Design review of the part shown in the three views and the two pictorial views. Dimensions are in mm from the part's minimum x, y and z. A direction names the side the tool comes from. Round coordinates to 2 decimals unless told otherwise and drop trailing zeros. Write each loop counter-clockwise with the first axis right and the second up, starting at its lowest first coordinate (ties: lowest second). Pieces come first, ordered by that corner, then holes. Notation, with made-up numbers: (-14, 49) - (33, 49) arc R6 cw to (33, 54) - close; hole circle Ø11 at (-23, 17.5). An arc over 180 degrees is marked (long way). One line per item, written item: value. Start each with the question number.
Q1. Clearance check with flat-ended pins moving along their axes: pin 1 Ø1.5 at (x, y) = (6.5, 1) entering from +Z; pin 2 Ø1 at (x, z) = (1.5, 3) entering from +Y; pin 3 Ø0.9 at (x, y) = (7.5, 2) entering from -Z; pin 4 Ø0.9 at (y, z) = (2, 1.5) entering from +X. State where each tip first meets the part, or that it passes through.
Q2. Mouldability with a two-part tool opening along X and no side actions: class the marked faces 4, 5, 6 and 7 as +X half, -X half, draft (parallel to the pull), parting line (faces both ways), or undercut.
Q3. Add section A-A on x = 4.2. Write out the cut boundary in (y, z), and give its area (3 significant figures).
Q4. Add section D-D on x = 1.5. Write out the cut boundary in (y, z).
Q5. Tool access review of the marked faces 1, 2 and 3: name each direction out of +Z, -Z, +X, -X, +Y, -Y from which nothing blocks a thin tool from reaching the whole face with its end or side.
Q6. Add section C-C on z = 12. Write out the cut boundary in (x, y), and give its area (3 significant figures).
Q7. Add section B-B on y = 1.15. Write out the cut boundary in (x, z).
Q8. For probe 1 along Z at (x, y) = (4.25, 1); probe 2 along Z at (x, y) = (6.5, 2.1); probe 3 along X at (y, z) = (1.65, 5), list the stretches that pass through material, from the lowest coordinate up.
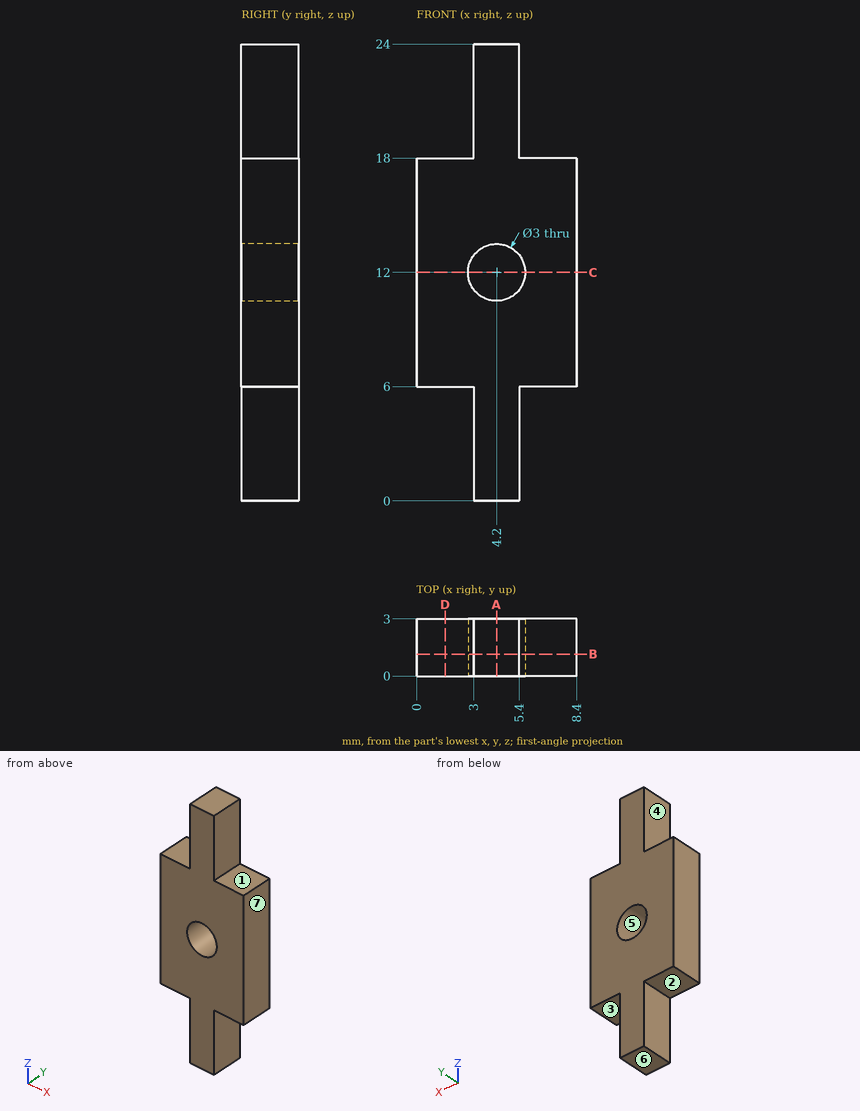
Result set:
1. pin 1: stops at z = 18
1. pin 2: passes through
1. pin 3: stops at z = 6
1. pin 4: stops at x = 5.4
2. face 4: -X half
2. face 5: undercut
2. face 6: draft
2. face 7: +X half
3. outline: (0, 0) - (3, 0) - (3, 10.5) - (0, 10.5) - close; (0, 13.5) - (3, 13.5) - (3, 24) - (0, 24) - close
3. area: 63.0 mm^2
4. outline: (0, 6) - (3, 6) - (3, 18) - (0, 18) - close
5. face 1: +Z, +X, +Y, -Y
5. face 2: -Z, -X, +Y, -Y
5. face 3: -Z, +X, +Y, -Y
6. outline: (0, 0) - (2.7, 0) - (2.7, 3) - (0, 3) - close; (5.7, 0) - (8.4, 0) - (8.4, 3) - (5.7, 3) - close
6. area: 16.2 mm^2
7. outline: (0, 6) - (3, 6) - (3, 0) - (5.4, 0) - (5.4, 6) - (8.4, 6) - (8.4, 18) - (5.4, 18) - (5.4, 24) - (3, 24) - (3, 18) - (0, 18) - close; hole circle Ø3 at (4.2, 12)
8. probe 1: z = 0 to 10.5, 13.5 to 24
8. probe 2: z = 6 to 18
8. probe 3: x = 3 to 5.4
